```python
from build123d import *

# Parameters (mm, degrees)
EXTRUDE_1_DEPTH          = 5
CUT_EXTRUDE_1_DEPTH      = 142.509716981
CUT_EXTRUDE_1_DEPTH_BACK = 142.509716981
HOLE_WIZARD_M5_1_D       = 4.2
HOLE_WIZARD_M3_1_D       = 2.5


with BuildPart() as part:
    # Sketch 1 → Extrude 1 (new body)
    with BuildSketch(Plane(origin=(0, 0, 0), x_dir=(1, 0, 0), z_dir=(0, 1, 0))):
        with BuildLine():
            Line((1.290175475, 43.716582347), (46.240484381, 88.666891252))
            ThreePointArc((46.240484381, 88.666891252), (6.697930583, -99.775436486), (-57.67661441, 81.690930648))
            ThreePointArc((-57.67661441, 81.690930648), (-51.783240076, 81.599208584), (-50.07196053, 75.95901388))
            ThreePointArc((-50.07196053, 75.95901388), (-37.241511516, 39.366784953), (1.290175475, 43.716582347))
        make_face()
        Polygon((8.361243287, 36.645514535), (43.716582347, 72.000853594), (40.181048441, 75.5363875), (4.825709381, 40.181048441), align=None, mode=Mode.SUBTRACT)
        with BuildLine():
            Line((-19.89891353, 23.499999452), (-19.898913286, 25.100000259))
            ThreePointArc((-19.898913286, 25.100000259), (-18.727340196, 27.92842699), (-15.898913286, 29.09999965))
            Line((-15.898913286, 29.09999965), (15.898913286, 29.09999965))
            ThreePointArc((15.898913286, 29.09999965), (18.727340196, 27.92842699), (19.898913286, 25.100000259))
            Line((19.898913286, 25.100000259), (19.89891353, 23.499999452))
            ThreePointArc((19.89891353, 23.499999452), (20.953647337, 20.953647337), (23.499999452, 19.89891353))
            Line((23.499999452, 19.89891353), (25.100000259, 19.898913286))
            ThreePointArc((25.100000259, 19.898913286), (27.92842699, 18.727340196), (29.09999965, 15.898913286))
            Line((29.09999965, 15.898913286), (29.09999965, -15.898913286))
            ThreePointArc((29.09999965, -15.898913286), (27.92842699, -18.727340196), (25.100000259, -19.898913286))
            Line((25.100000259, -19.898913286), (23.499999452, -19.89891353))
            ThreePointArc((23.499999452, -19.89891353), (20.953647337, -20.953647337), (19.89891353, -23.499999452))
            Line((19.89891353, -23.499999452), (19.898913286, -25.100000259))
            ThreePointArc((19.898913286, -25.100000259), (18.727340196, -27.92842699), (15.898913286, -29.09999965))
            Line((15.898913286, -29.09999965), (-15.898913286, -29.09999965))
            ThreePointArc((-15.898913286, -29.09999965), (-18.727340196, -27.92842699), (-19.898913286, -25.100000259))
            Line((-19.898913286, -25.100000259), (-19.89891353, -23.499999452))
            ThreePointArc((-19.89891353, -23.499999452), (-20.953647337, -20.953647337), (-23.499999452, -19.89891353))
            Line((-23.499999452, -19.89891353), (-25.100000259, -19.898913286))
            ThreePointArc((-25.100000259, -19.898913286), (-27.92842699, -18.727340196), (-29.09999965, -15.898913286))
            Line((-29.09999965, -15.898913286), (-29.09999965, 15.898913286))
            ThreePointArc((-29.09999965, 15.898913286), (-27.92842699, 18.727340196), (-25.100000259, 19.898913286))
            Line((-25.100000259, 19.898913286), (-23.499999452, 19.89891353))
            ThreePointArc((-23.499999452, 19.89891353), (-20.953647337, 20.953647337), (-19.89891353, 23.499999452))
        make_face(mode=Mode.SUBTRACT)
        Polygon((-43.716582347, -72.000853594), (-40.181048441, -75.5363875), (-4.825709381, -40.181048441), (-8.361243287, -36.645514535), align=None, mode=Mode.SUBTRACT)
    extrude(amount=-EXTRUDE_1_DEPTH)

    # Sketch 5 → Cut-Extrude 1 (cut, two sides: drawn at the far end of the back side and taken through both)
    with BuildSketch(Plane(origin=(0, 0, 0), x_dir=(1, 0, 0), z_dir=(0, 1, 0)).offset(-CUT_EXTRUDE_1_DEPTH_BACK)):
        with BuildLine():
            Line((-34.09999965, -5), (-34.09999965, 5))
            ThreePointArc((-34.09999965, 5), (-29.09999965, 10), (-24.09999965, 5))
            Line((-24.09999965, 5), (-24.09999965, -5))
            ThreePointArc((-24.09999965, -5), (-29.09999965, -10), (-34.09999965, -5))
        make_face()
    extrude(amount=CUT_EXTRUDE_1_DEPTH + CUT_EXTRUDE_1_DEPTH_BACK, mode=Mode.SUBTRACT)

    # Hole Wizard M5 _1 (through all)
    with Locations(Plane(origin=(0, 0, 0), x_dir=(1, 0, 0), z_dir=(0, 1, 0))):
        with Locations((23.5, 23.5), (23.5, -23.5), (-23.5, -23.5), (-23.5, 23.5)):
            Hole(HOLE_WIZARD_M5_1_D / 2)

    # Hole Wizard M3 _1 (through all)
    with Locations(Plane(origin=(0, 0, 0), x_dir=(1, 0, 0), z_dir=(0, 1, 0))):
        with Locations((-69.282032303, 40), (0, -80), (69.282032303, 40)):
            Hole(HOLE_WIZARD_M3_1_D / 2)


solid = part.part
```
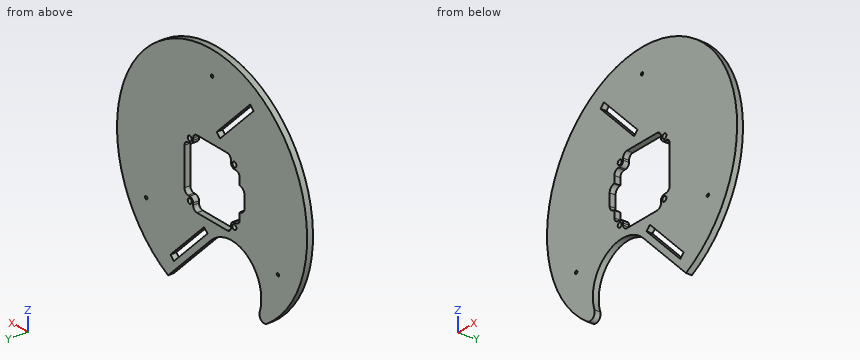
Check sheet for the modelled part. Datum: model origin and axes. Units: mm. Coordinates: 2 decimals unless noted, no trailing zeros. Loops run counter-clockwise (first coordinate to the right, second up) from the corner with the lowest first, then second, coordinate; pieces in that order, holes last. Notation, with made-up numbers: M 59,-14.75 L 79,-14.75 A26 ccw 79,8.25 Z; hole C 78.25,-13 d8. An arc over 180 degrees is marked long. Answer as a JSON object with one key per item and string values.
1. Sectioned sample at B-B on y = -2.55. Count the separate pieces of the cut face and the enclosed holes in it, and give its area (3 significant figures).
Outcome:
{"separate pieces": "1", "enclosed holes": "10", "area": "23,400 mm²"}
2. Sectioned sample at A-A on z = 0. Record the cut outline in (x, y).
Outcome:
{"outline": "M -100,-5 L -34.1,-5 L -34.1,0 L -100,0 Z; M 29.1,-5 L 100,-5 L 100,0 L 29.1,0 Z"}
3. Scan lines: L1, parallel to X at y = -0.4, z = -1.5; L2, parallel to X at y = -3.4, z = 3; L3, parallel to X at y = -2.95, z = -40. Record each from-to range of solid material in increasing order. Write a range as from..to.
Outcome:
{"L1": "-99.99..-34.1, 29.1..99.99", "L2": "-99.95..-34.1, 29.1..99.95", "L3": "-91.65..-70.53, -68.03..-38.21, -3.2..5.01, 11.72..68.03, 70.53..91.65"}
4. Depth check by flat-ended pin: P1, Ø0.8, axis at x = -24, y = -3.5, coming from the -Z side; P2, Ø0.8, axis at y = -2, z = 24.5, coming from the +X side; P3, Ø1.3, axis at y = -3, z = 24.5, coming from the -X side; P4, Ø6.5, axis at x = 23.5, z = 23.5, coming from the +Y side. Enter the tip coordinate at first touch or a pass-through.
Outcome:
{"P1": "z = -34.83", "P2": "x = 97.05", "P3": "x = -97.11", "P4": "y = 0"}
